from build123d import *

# Parameters (mm, degrees)
F0_W      = 72.000258
F0_H      = 78.241773
F1_DEPTH  = 228.6
F3_DEPTH  = 25.4
F4_R      = 21.565996
F5_DEPTH  = 177.8
F6_R      = 13.479232
F7_DEPTH  = 76.2
F8_W      = 23.628573
F8_H      = 50.823714
F9_DEPTH  = 1778
F11_DEPTH = 177.8


with BuildPart() as f1:
    # F0 (on Top) → F1 (new body)
    with BuildSketch(Plane.XY):
        with Locations((36.000129, -39.120886)):
            Rectangle(F0_W, F0_H)
    extrude(amount=F1_DEPTH)

    # F2 (on face) → F3 (join)
    with BuildSketch(Plane(origin=(0, 0, 0), x_dir=(0, -1, 0), z_dir=(-1, 0, 0))):
        Polygon((59.31577, 109.609046), (52.362666, 120.328418), (40.436798, 124.913641), (28.093442, 121.613314), (20.04734, 111.688051), (19.371831, 98.928965), (26.324935, 88.209593), (38.250803, 83.62437), (50.594159, 86.924697), (58.64026, 96.84996), align=None)
    extrude(amount=F3_DEPTH)

    # F4 (on face) → F5 (cut)
    with BuildSketch(Plane.XY.offset(228.6)):
        with Locations((33.99393, -39.343797)):
            Circle(F4_R)
    extrude(amount=-F5_DEPTH, mode=Mode.SUBTRACT)

    # F6 (on face) → F7 (cut)
    with BuildSketch(Plane(origin=(-25.4, 0, 0), x_dir=(0, -1, 0), z_dir=(-1, 0, 0))):
        with Locations((38.675066, 103.229503)):
            Circle(F6_R)
    extrude(amount=-F7_DEPTH, mode=Mode.SUBTRACT)

    # F8 (on face) → F9 (join)
    with BuildSketch(Plane.YZ.offset(72.000258)):
        with Locations((-54.278838, 87.327758)):
            Rectangle(F8_W, F8_H)
    extrude(amount=F9_DEPTH)

    # F10 (on face) → F11 (join)
    with BuildSketch(Plane(origin=(0, 0, 0), x_dir=(0, -1, 0), z_dir=(-1, 0, 0))):
        Polygon((38.63069, 56.816015), (31.828527, 56.816015), (25.614442, 54.049327), (21.062907, 48.994335), (18.960923, 42.525093), (19.671943, 35.760194), (23.073024, 29.869348), (28.576089, 25.871137), (35.229608, 24.456888), (41.883128, 25.871137), (47.386193, 29.869348), (50.787274, 35.760194), (51.498294, 42.525093), (49.39631, 48.994335), (44.844775, 54.049327), align=None)
    extrude(amount=F11_DEPTH)


solid = f1.part
For this review, take the finished solid that the model builds, in its own axes (mm). A direction names the side the tool comes from. Coordinates: 2 decimals unless noted, no trailing zeros. Loops run counter-clockwise (first coordinate to the right, second up) from the corner with the lowest first, then second, coordinate; pieces in that order, holes last. Notation, with made-up numbers: (-6.5, -27.5) - (46.5, -27.5) arc R19 ccw to (46.5, -3.5) - close; hole circle Ø7 at (-7.75, 16.5). An arc over 180 degrees is marked (long way). Use a Markdown table: item, result. Add a question column.
Item 1: Insertion check: pin 1 Ø12 at (y, z) = (-33.5, 113) entering from -X; pin 2 Ø2 at (x, y) = (-123.5, -34.5) entering from +Z; pin 3 Ø6 at (x, z) = (452.5, 63.5) entering from +Y. Each pin has a flat end and moves straight along its axis. Give the tip position at first contact, or say it passes through.
Item 2: We need section A-A (z = 168.5). Give the boundary of the cut face in (x, y), and give its area (3 significant figures).
Item 3: For line 1 (X direction, y = -12.5, z = 22.5); line 2 (Y direction, x = 1650.5, z = 109); line 3 (X direction, y = -42, z = 44.5), list the stretches that pass through material, from the lowest coordinate up.
Item 4: We need section B-B (x = 1263.5). Give the boundary of the cut face in (y, z).
Item 5: Mouldability with a two-part tool opening along X and no side actions: class faces 5 (the face through (0, -40, 138)), 6 (the face through (34, -39, 50.8)), 7 (the face through (51, -21, 228.6)) as pulls with the +X half, pulls with the -X half, needs draft (parallel to the pull), parting line crosses it, or undercut.
Item 6: Tool access review of faces 1 (the face through (-25.4, -48, 114)), 2 (the face through (53.915, -47.604, 140.945)), 3 (the face through (949, -42.465, 87)), 4 (the face through (949, -66.093, 87)): name each direction out of +Z, -Z, +X, -X, +Y, -Y from which nothing blocks a thin tool from reaching the whole face with its end or side.
Results list:
| question | item | result |
|---|---|---|
| 1 | pin 1 | stops at x = -25.4 |
| 1 | pin 2 | stops at z = 56.82 |
| 1 | pin 3 | stops at y = -42.46 |
| 2 | outline | (0, -78.24) - (72, -78.24) - (72, 0) - (0, 0) - close; hole circle Ø43.13 at (33.99, -39.34) |
| 2 | area | 4,170 mm^2 |
| 3 | line 1 | x = 0 to 72 |
| 3 | line 2 | y = -66.09 to -42.46 |
| 3 | line 3 | x = -177.8 to 72 |
| 4 | outline | (-66.09, 61.92) - (-42.46, 61.92) - (-42.46, 112.74) - (-66.09, 112.74) - close |
| 5 | face 5 | pulls with the -X half |
| 5 | face 6 | undercut |
| 5 | face 7 | needs draft |
| 6 | face 1 | +Z, -X, +Y, -Y |
| 6 | face 2 | +Z |
| 6 | face 3 | +Z, -Z, +X, +Y |
| 6 | face 4 | +Z, -Z, +X, -Y |
